Part model, mm, in its own coordinate system. Face numbers are marked on the shaded views. A direction names the side the tool comes from. Give positions to 0.01 mm unless a question says otherwise; leave off trailing zeros. Write each loop counter-clockwise with the first axis right and the second up, starting at its lowest first coordinate (ties: lowest second). Pieces come first, ordered by that corner, then holes. Notation, with made-up numbers: M 43.5,42.25 L 56.5,42.25 A17 cw 56.5,64.25 Z; hole C 13.25,-35.5 d9. An arc over 180 degrees is marked long. Use CSV: the item, a comma, the result in double quotes. Start each with the question number.
Item 1: Drill centre lines: line 1 (Y direction, x = 0, z = 4.6); line 2 (X direction, y = 6.5, z = 1); line 3 (X direction, y = 24, z = 4). Where is each one in solid material? Low to high. Write a range as [from, to].
Item 2: Which spindle directions (+Z, -Z, +X, -X, +Y, -Y) get a long thin tool onto all of the face, cutting with end or side? Do the marked faces 1, 2, 3, 4 and 5. Say none if no direction does.
Item 3: Pin check, flat tips, straight feed: pin 1 (1.8 mm diameter, centred on y = -5.5, z = 2, fed in from -X); pin 2 (3 mm diameter, centred on y = -3, z = 2, fed in from +X); pin 3 (2.5 mm diameter, centred on x = -5.5, y = -6, fed in from -Z). Stop position of each tip, or through.
Item 4: Cut at C-C (z = 2). Count the separate pieces of the cut face and the enclosed holes in it, then the cut area to 3 significant figures.
Item 5: Cut at A-A (x = 0). List the corners of the cut face in (y, z), then the cut area to 3 significant figures.
Item 6: Mould opens along Z. For the marked faces 6, 7 and 8 say: released by +Z, released by -Z, zero draft, split by the parting line, or undercut.
Item 7: Cut at D-D (x = -5.5). List the corners of the cut face in (y, z).
Item 8: Cut at B-B (y = 20). List the corners of the cut face in (x, z).
from build123d import *

# Parameters (mm, degrees)
SKETCH_1_R               = 7.5
EXTRUDE_1_DEPTH          = 6
FILLET_1_R               = 10
SKETCH_2_R               = 1.5
SKETCH_2_R_2             = 3
CUT_EXTRUDE_1_DEPTH      = 3.5
CUT_EXTRUDE_2_DEPTH      = 29.957943642
CUT_EXTRUDE_2_DEPTH_BACK = 29.957943642
SKETCH_3_R               = 1.5
CUT_EXTRUDE_3_DEPTH      = 30.365157926
CUT_EXTRUDE_3_DEPTH_BACK = 2.5
CUT_EXTRUDE_START        = -5
CUT_EXTRUDE_4_DEPTH      = 5
CUT_EXTRUDE_5_DEPTH      = 31.10087208
CUT_EXTRUDE_5_DEPTH_BACK = 31.10087208
SKETCH_6_R               = 1
CUT_EXTRUDE_6_DEPTH      = 31.1008721
CUT_EXTRUDE_6_DEPTH_BACK = 31.1008721
SKETCH_7_R               = 1


# Read off the part's stored shape, not the designer's step: 除料-伸長4
with BuildPart() as part:
    # 草圖1 → 填料-伸長1 (new body)
    with BuildSketch(Plane.XY):
        Circle(SKETCH_1_R)
        with BuildLine():
            Line((-3.75, 0), (-3.75, 24))
            ThreePointArc((-3.75, 24), (0, 27.75), (3.75, 24))
            Line((3.75, 24), (3.75, 0))
            ThreePointArc((3.75, 0), (0, -3.75), (-3.75, 0))
        make_face()
    extrude(amount=EXTRUDE_1_DEPTH)

    # 圓角1
    fillet_1_edges = [part.edges().sort_by_distance(p)[0] for p in [
        (-3.75, 6.495190528, 3),
        (3.75, 6.495190528, 3),
    ]]
    fillet(fillet_1_edges, radius=FILLET_1_R)

    # 草圖2 → 除料-伸長1 (cut)
    with BuildSketch(Plane(origin=(0, 0, 0), x_dir=(-1, 0, 0), z_dir=(0, 0, -1))):
        with Locations((0, 24)):
            Circle(SKETCH_2_R)
        Circle(SKETCH_2_R_2)
    extrude(amount=-CUT_EXTRUDE_1_DEPTH, mode=Mode.SUBTRACT)

    # 草圖3 → 除料-伸長2 (cut, two sides: drawn at the far end of the back side and taken through both)
    with BuildSketch(Plane(origin=(0, 0, 3.5), x_dir=(-1, 0, 0), z_dir=(0, 0, -1)).offset(-CUT_EXTRUDE_2_DEPTH_BACK)):
        with BuildLine():
            Line((-0.5, 7.585786438), (-0.5, 1.414213562))
            ThreePointArc((-0.5, 1.414213562), (-1.5, 0), (-0.5, -1.414213562))
            Line((-0.5, -1.414213562), (-0.5, -8))
            ThreePointArc((-0.5, -8), (0, -8.5), (0.5, -8))
            Line((0.5, -8), (0.5, -1.414213562))
            ThreePointArc((0.5, -1.414213562), (1.5, 0), (0.5, 1.414213562))
            Line((0.5, 1.414213562), (0.5, 7.585786438))
            ThreePointArc((0.5, 7.585786438), (0, 10.5), (-0.5, 7.585786438))
        make_face()
        with Locations((0, 24)):
            Circle(SKETCH_3_R)
        with Locations((0, 20)):
            Circle(SKETCH_3_R)
    extrude(amount=CUT_EXTRUDE_2_DEPTH + CUT_EXTRUDE_2_DEPTH_BACK, mode=Mode.SUBTRACT)

    # 草圖4 → 除料-伸長3 (cut, two sides: drawn at the far end of the back side and taken through both)
    with BuildSketch(Plane(origin=(0, 0, 0), x_dir=(-1, 0, 0), z_dir=(0, 0, -1)).offset(-CUT_EXTRUDE_3_DEPTH_BACK)):
        with BuildLine():
            Line((0.5, 7.585786438), (0.5, 7.483314774))
            ThreePointArc((0.5, 7.483314774), (3.498440712, 6.634072097), (5.892857143, 4.639421806))
            ThreePointArc((5.892857143, 4.639421806), (4.300888175, 7.552049194), (3.75, 10.825317547))
            Line((3.75, 10.825317547), (3.75, 24))
            ThreePointArc((3.75, 24), (0, 27.75), (-3.75, 24))
            Line((-3.75, 24), (-3.75, 10.825317547))
            ThreePointArc((-3.75, 10.825317547), (-4.300888175, 7.552049194), (-5.892857143, 4.639421806))
            ThreePointArc((-5.892857143, 4.639421806), (-3.498440712, 6.634072097), (-0.5, 7.483314774))
            Line((-0.5, 7.483314774), (-0.5, 7.585786438))
            ThreePointArc((-0.5, 7.585786438), (0, 10.5), (0.5, 7.585786438))
        make_face()
        with BuildLine():
            ThreePointArc((-2.656851136, 23.290322581), (0, 26.75), (2.656851136, 23.290322581))
            ThreePointArc((2.656851136, 23.290322581), (2.487489566, 22), (2.656851136, 20.709677419))
            ThreePointArc((2.656851136, 20.709677419), (0, 17.25), (-2.656851136, 20.709677419))
            ThreePointArc((-2.656851136, 20.709677419), (-2.487489566, 22), (-2.656851136, 23.290322581))
        make_face(mode=Mode.SUBTRACT)
    extrude(amount=CUT_EXTRUDE_3_DEPTH + CUT_EXTRUDE_3_DEPTH_BACK, mode=Mode.SUBTRACT)

    # 除料-伸長4 outline → 除料-伸長4 (cut)
    with BuildSketch(Plane(origin=(0, 0, 0), x_dir=(-1, 0, 0), z_dir=(0, 0, -1)).offset(CUT_EXTRUDE_START)):
        with BuildLine():
            ThreePointArc((-4.090898557, 8.23654191), (-4.80910956, 6.346425035), (-5.892857143, 4.639421806))
            ThreePointArc((-5.892857143, 4.639421806), (-6.569636137, 3.617994061), (-7.071067812, 2.5))
            Line((-7.071067812, 2.5), (-3.5, 2.5))
            ThreePointArc((-3.5, 2.5), (-2.792893219, 2.792893219), (-2.5, 3.5))
            Line((-2.5, 3.5), (-2.5, 7.071067812))
            ThreePointArc((-2.5, 7.071067812), (-3.250743509, 7.714829249), (-4.090898557, 8.23654191))
        make_face()
        with BuildLine():
            Line((7.071067812, -2.5), (3.5, -2.5))
            ThreePointArc((3.5, -2.5), (2.792893219, -2.792893219), (2.5, -3.5))
            Line((2.5, -3.5), (2.5, -7.071067812))
            ThreePointArc((2.5, -7.071067812), (5.303300859, -5.303300859), (7.071067812, -2.5))
        make_face()
    extrude(amount=CUT_EXTRUDE_4_DEPTH, mode=Mode.SUBTRACT)

    # 草圖6 → 除料-伸長5 (cut, two sides: drawn at the far end of the back side and taken through both)
    with BuildSketch(Plane.ZY.offset(2.5).offset(-CUT_EXTRUDE_5_DEPTH_BACK)):
        with Locations((2, -5.071067812)):
            Circle(SKETCH_6_R)
    extrude(amount=CUT_EXTRUDE_5_DEPTH + CUT_EXTRUDE_5_DEPTH_BACK, mode=Mode.SUBTRACT)

    # 草圖7 → 除料-伸長6 (cut, two sides: drawn at the far end of the back side and taken through both)
    with BuildSketch(Plane(origin=(2.5, 0, 0), x_dir=(0, 0, -1), z_dir=(1, 0, 0)).offset(-CUT_EXTRUDE_6_DEPTH_BACK)):
        with Locations(Location((-2, 5.483314774, 0), (0, 0, 90))):
            Circle(SKETCH_7_R)
    extrude(amount=CUT_EXTRUDE_6_DEPTH + CUT_EXTRUDE_6_DEPTH_BACK, mode=Mode.SUBTRACT)


solid = part.part
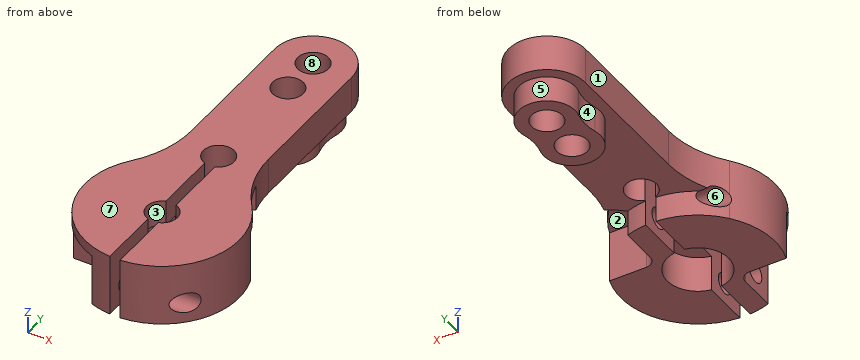
Worked answers:
1,line 1,"y = [10.5, 18.5], [21.5, 22.5], [25.5, 27.75]"
1,line 2,"x = [-3.74, -0.5], [0.5, 2.5]"
1,line 3,"x = [-3.75, -1.5], [1.5, 3.75]"
2,face 1,"+Z, -Z, -X, +Y"
2,face 2,"-Z, +X"
2,face 3,"+Z, -Z"
2,face 4,"-Z, -X"
2,face 5,"-Z"
3,pin 1,"stops at x = -2.5"
3,pin 2,"stops at x = 7.35"
3,pin 3,"stops at z = 5"
4,separate pieces,"7"
4,enclosed holes,"2"
4,area,"116 mm^2"
5,outline,"M 10.5,2.5 L 17.25,2.5 L 17.25,0 L 18.5,0 L 18.5,6 L 10.5,6 Z; M 21.5,0 L 22.5,0 L 22.5,6 L 21.5,6 Z; M 25.5,0 L 26.75,0 L 26.75,2.5 L 27.75,2.5 L 27.75,6 L 25.5,6 Z"
5,area,"48.1 mm^2"
6,face 6,"undercut"
6,face 7,"released by +Z"
6,face 8,"zero draft"
7,outline,"M -5.1,5 L -2.5,5 L -2.5,0 L 5.1,0 L 5.1,1.08 A1 cw 5.17,2.95 L 5.17,6 L -5.1,6 Z"
8,outline,"M -3.75,2.5 L -2.75,2.5 L -2.75,0 L -1.5,0 L -1.5,6 L -3.75,6 Z; M 1.5,0 L 2.75,0 L 2.75,2.5 L 3.75,2.5 L 3.75,6 L 1.5,6 Z"
